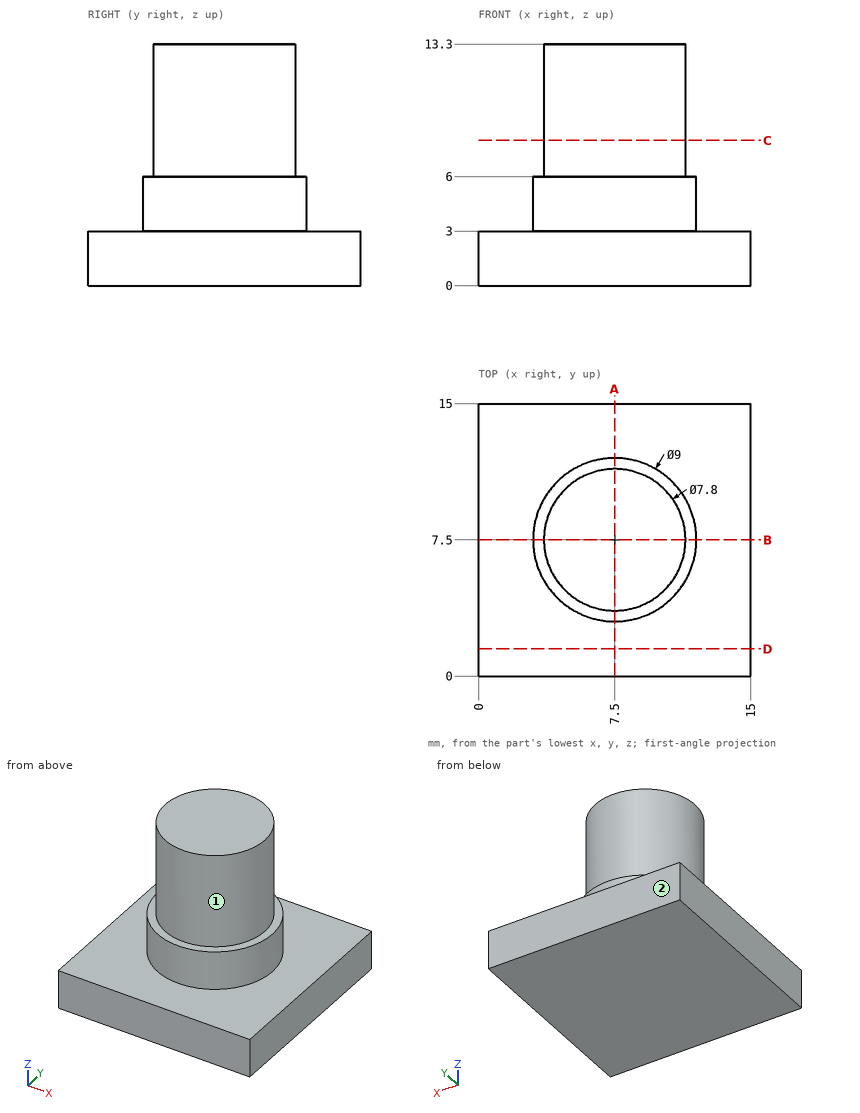
Part print with two shaded views. Sizes in mm from the minimum x, y, z corner. A direction names the side the tool comes from. Coordinates: 2 decimals unless noted, no trailing zeros. Order: outer loops, then holes, each group sorted by start corner. A loop starts at its lowest first (then second) coordinate and runs counter-clockwise, first axis right, second up. Notation, with made-up numbers: M 42.25,84 L 73.25,84 A22 cw 73.25,122 Z; hole C 62,61 d6. An arc over 180 degrees is marked long. Use a Markdown table: item, result.
(1) Tool access for the marked faces 1 and 2: list every direction of +Z, -Z, +X, -X, +Y, -Y with a clear straight run to the whole face (end or side of a thin tool).
A:
| item | result |
|---|---|
| face 1 | +Z |
| face 2 | +Z, -Z, +X, -X, +Y |
(2) Probe L1, parallel to Z at x = 0.5, y = 1; L2, parallel to X at y = 9, z = 3.5; L3, parallel to Y at x = 4.5, z = 8. List the from-to ranges inside material, lowest first.
A:
| item | result |
|---|---|
| L1 | z = 0 to 3 |
| L2 | x = 3.26 to 11.74 |
| L3 | y = 5.01 to 9.99 |
(3) Flat gauge pin, fed straight in: pin 1 (2 mm diameter, centred on y = 4.5, z = 9, fed in from +X). Where does the tip first touch, or does it go through?
A:
| item | result |
|---|---|
| pin 1 | stops at x = 10.85 |
(4) Cut at D-D on y = 1.5. Write the cut outline in (x, z), then the cut area to 3 significant figures.
A:
| item | result |
|---|---|
| outline | M 0,0 L 15,0 L 15,3 L 0,3 Z |
| area | 45.0 mm^2 |
(5) Cut at C-C on z = 8. Write the cut outline in (x, y).
A:
| item | result |
|---|---|
| outline | C 7.5,7.5 d7.8 |
(6) Cut at A-A on x = 7.5. Write the cut outline in (y, z), then the cut area to 3 significant figures.
A:
| item | result |
|---|---|
| outline | M 0,0 L 15,0 L 15,3 L 12,3 L 12,6 L 11.4,6 L 11.4,13.3 L 3.6,13.3 L 3.6,6 L 3,6 L 3,3 L 0,3 Z |
| area | 129 mm^2 |
